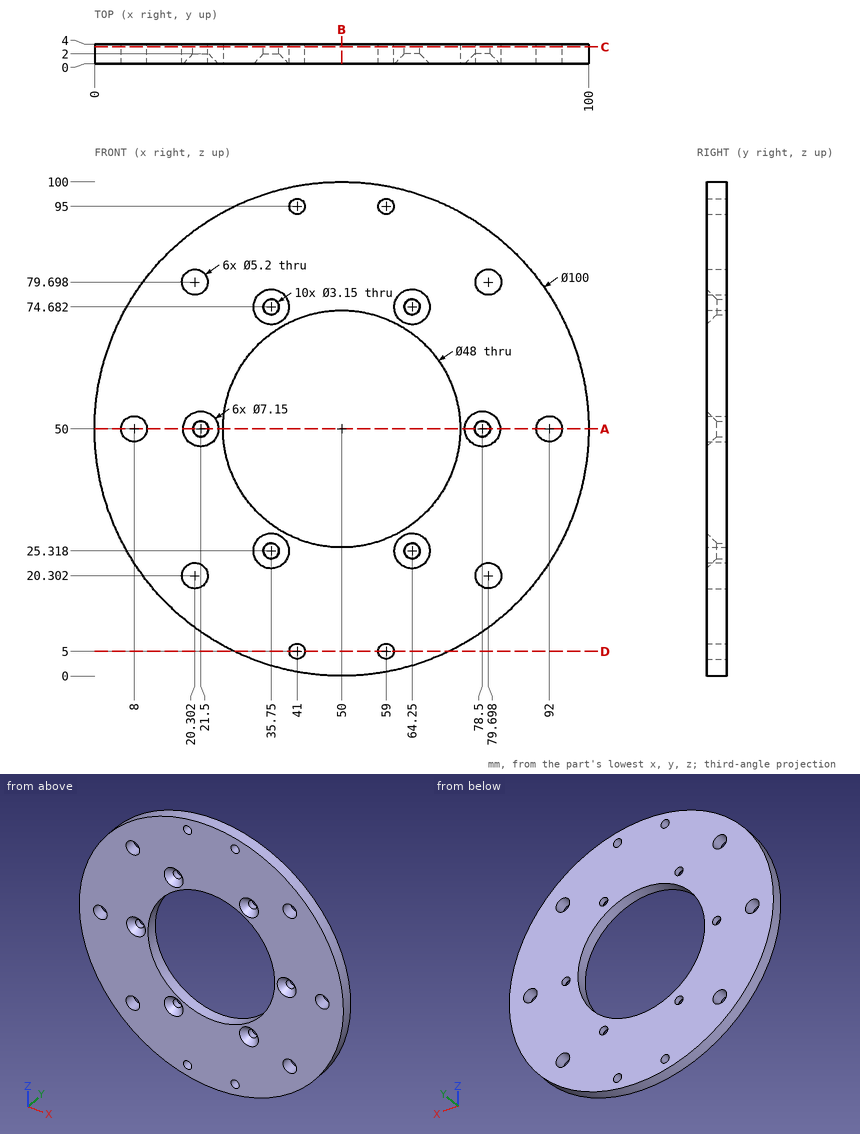
Here's the drawing with two shaded views (mm, measured from the low corner). I have some questions. Coordinates: 2 decimals unless noted, no trailing zeros. Order: outer loops, then holes, each group sorted by start corner. A loop starts at its lowest first (then second) coordinate and runs counter-clockwise, first axis right, second up. Notation, with made-up numbers: (-15, 28.25) - (30, 28.25) arc R20 cw to (30, 42.25) - close; hole circle Ø5 at (-1.5, 57.25). An arc over 180 degrees is marked (long way). Use CSV: the item, a comma, the result in double quotes. Start each with the question number.
1. Suppose I cut it at B-B on x = 50. List the corners of the cut face in (y, z) for me.
2. Suppose I cut it at C-C on y = 3.4. Give the number of separate pieces and of enclosed holes in the cut face, then the cut area to 3 significant figures.
3. Suppose I cut it at D-D on z = 5. List the corners of the cut face in (x, y) for me (1 decimal).
4. Suppose I cut it at A-A on z = 50. List the corners of the cut face in (x, y) for me (1 decimal), then the cut area to 3 significant figures.
5. Please list where these lines run through material, in increasing order: line 1 (X direction, y = 2.7, z = 50) (1 decimal); line 2 (Z direction, x = 49, y = 1.4); line 3 (Z direction, x = 42, y = 0.3) (1 decimal). Write a range as from..to.
6. I'm going to push flat-ended pins straight in: pin 1 (1.5 mm diameter, centred on x = 66.5, y = 2.5, fed in from +Z) (1 decimal); pin 2 (1 mm diameter, centred on x = 80, y = 3, fed in from -Z); pin 3 (1 mm diameter, centred on x = 68, y = 1, fed in from -Z). Where does each tip first touch, or does it pass through?
Output:
1,outline,"(0, 0) - (4, 0) - (4, 26) - (0, 26) - close; (0, 74) - (4, 74) - (4, 100) - (0, 100) - close"
2,separate pieces,"1"
2,enclosed holes,"17"
2,area,"5,840 mm2"
3,outline,"(28.2, 0) - (39.4, 0) - (39.4, 4) - (28.2, 4) - close; (42.6, 0) - (57.4, 0) - (57.4, 4) - (42.6, 4) - close; (60.6, 0) - (71.8, 0) - (71.8, 4) - (60.6, 4) - close"
4,outline,"(0, 0) - (5.4, 0) - (5.4, 4) - (0, 4) - close; (10.6, 0) - (17.9, 0) - (19.9, 2) - (19.9, 4) - (10.6, 4) - close; (23.1, 2) - (25.1, 0) - (26, 0) - (26, 4) - (23.1, 4) - close; (74, 0) - (74.9, 0) - (76.9, 2) - (76.9, 4) - (74, 4) - close; (80.1, 2) - (82.1, 0) - (89.4, 0) - (89.4, 4) - (80.1, 4) - close; (94.6, 0) - (100, 0) - (100, 4) - (94.6, 4) - close"
4,area,"133 mm2"
5,line 1,"x = 0..5.4, 10.6..19.9, 23.1..26, 74..76.9, 80.1..89.4, 94.6..100"
5,line 2,"z = 0.01..26.02, 73.98..99.99"
5,line 3,"z = 0.6..3.8, 6.2..27.4, 72.6..93.8, 96.2..99.4"
6,pin 1,"stops at z = 97.5"
6,pin 2,"stops at z = 9.63"
6,pin 3,"stops at z = 3.16"
